Build history of the part. All positions in model axes, mm. Face numbers are marked on the shaded views. A direction names the side the tool comes from. Round coordinates to 2 decimals unless told otherwise and drop trailing zeros. Loops run counter-clockwise (first coordinate to the right, second up) from the corner with the lowest first, then second, coordinate; pieces in that order, holes last.
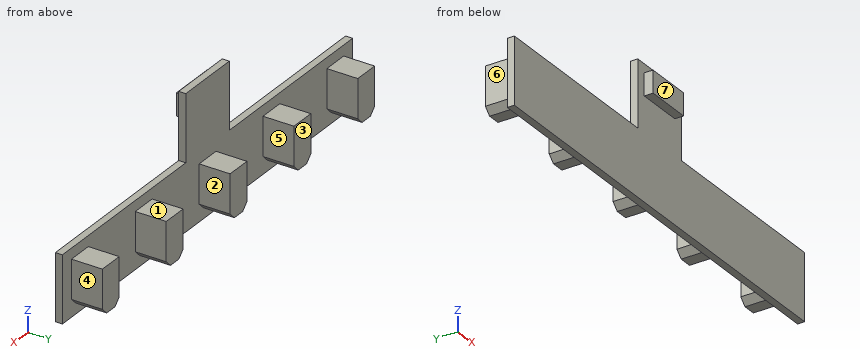
from build123d import *

# Parameters (mm, degrees)
SKETCH1_W           = 15
SKETCH1_H           = 15
SKETCH1_W_2         = 10.56
SKETCH1_H_2         = 5
BOSS_EXTRUDE1_DEPTH = 1.6
SKETCH1_3_W         = 10.56
SKETCH1_3_H         = 5
BOSS_EXTRUDE2_DEPTH = 2
BOSS_EXTRUDE3_DEPTH = 8.6


with BuildPart() as part:
    # Sketch1 → Boss-Extrude1 (new body)
    # profile 1 of 3: a face of its own
    with BuildSketch(Plane(origin=(0, 0, 0), x_dir=(1, 0, 0), z_dir=(0, 1, 0))):
        with Locations((0, 3)):
            Rectangle(SKETCH1_W, SKETCH1_H)
        Rectangle(SKETCH1_W_2, SKETCH1_H_2, mode=Mode.SUBTRACT)
    # profile 2 of 3: a face of its own
    with BuildSketch(Plane(origin=(0, 0, 0), x_dir=(1, 0, 0), z_dir=(0, 1, 0))):
        Rectangle(SKETCH1_W_2, SKETCH1_H_2)
    # profile 3 of 3: a face of its own
    with BuildSketch(Plane(origin=(0, 0, 0), x_dir=(1, 0, 0), z_dir=(0, 1, 0))):
        Polygon((-50, 10.5), (-7.5, 10.5), (7.5, 10.5), (50, 10.5), (50, 25.5), (-50, 25.5), align=None)
        Polygon((-42.569302237, 23.1), (-41.1, 21.630697763), (-41.1, 12.9), (-46.9, 12.9), (-46.9, 21.630697763), (-45.430697763, 23.1), align=None, mode=Mode.SUBTRACT)
        Polygon((-20.569302237, 23.1), (-19.1, 21.630697763), (-19.1, 12.9), (-24.9, 12.9), (-24.9, 21.630697763), (-23.430697763, 23.1), align=None, mode=Mode.SUBTRACT)
        Polygon((2.9, 12.9), (-2.9, 12.9), (-2.9, 21.630697763), (-1.430697763, 23.1), (1.430697763, 23.1), (2.9, 21.630697763), align=None, mode=Mode.SUBTRACT)
        Polygon((23.430697763, 23.1), (24.9, 21.630697763), (24.9, 12.9), (19.1, 12.9), (19.1, 21.630697763), (20.569302237, 23.1), align=None, mode=Mode.SUBTRACT)
        Polygon((45.430697763, 23.1), (46.9, 21.630697763), (46.9, 12.9), (41.1, 12.9), (41.1, 21.630697763), (42.569302237, 23.1), align=None, mode=Mode.SUBTRACT)
    extrude(amount=BOSS_EXTRUDE1_DEPTH)

    # Sketch1_3 → Boss-Extrude2 (add)
    with BuildSketch(Plane(origin=(0, 0, 0), x_dir=(1, 0, 0), z_dir=(0, 1, 0))):
        Rectangle(SKETCH1_3_W, SKETCH1_3_H)
    extrude(amount=-BOSS_EXTRUDE2_DEPTH)

    # Sketch1_4 → Boss-Extrude3 (add)
    with BuildSketch(Plane(origin=(0, 0, 0), x_dir=(1, 0, 0), z_dir=(0, 1, 0))):
        Polygon((23.430697763, 23.1), (24.9, 21.630697763), (24.9, 12.9), (19.1, 12.9), (19.1, 21.630697763), (20.569302237, 23.1), align=None)
        Polygon((45.430697763, 23.1), (46.9, 21.630697763), (46.9, 12.9), (41.1, 12.9), (41.1, 21.630697763), (42.569302237, 23.1), align=None)
        Polygon((2.9, 21.630697763), (2.9, 12.9), (-2.9, 12.9), (-2.9, 21.630697763), (-1.430697763, 23.1), (1.430697763, 23.1), align=None)
        Polygon((-20.569302237, 23.1), (-19.1, 21.630697763), (-19.1, 12.9), (-24.9, 12.9), (-24.9, 21.630697763), (-23.430697763, 23.1), align=None)
        Polygon((-42.569302237, 23.1), (-41.1, 21.630697763), (-41.1, 12.9), (-46.9, 12.9), (-46.9, 21.630697763), (-45.430697763, 23.1), align=None)
    extrude(amount=BOSS_EXTRUDE3_DEPTH)


solid = part.part
(1) Which spindle directions (+Z, -Z, +X, -X, +Y, -Y) get a long thin tool onto all of the face, cutting with end or side? Do the marked faces 1, 2 and 3. Say none if no direction does.
Responses:
face 1: +Z, +X, -X, +Y
face 2: +Z, -Z, +Y
face 3: +Z, -Z, +X, -X, +Y
(2) Probe line 1 (X direction, y = 2.75, z = -14.25); line 2 (X direction, y = 7.5, z = -22.5); line 3 (Y direction, x = 11, z = -11.75). List the from-to ranges inside material, lowest first.
Responses:
line 1: x = -46.9 to -41.1, -24.9 to -19.1, -2.9 to 2.9, 19.1 to 24.9, 41.1 to 46.9
line 2: x = -46.03 to -41.97, -24.03 to -19.97, -2.03 to 2.03, 19.97 to 24.03, 41.97 to 46.03
line 3: y = 0 to 1.6
(3) Slice it at C-C on y = -1. List the corners of the cut face in (x, z), plus the area to 3 significant figures.
Responses:
outline: (-5.28, -2.5) - (5.28, -2.5) - (5.28, 2.5) - (-5.28, 2.5) - close
area: 52.8 mm2
(4) Slice it at B-B on z = -15.5. List the corners of the cut face in (x, y).
Responses:
outline: (-50, 0) - (50, 0) - (50, 1.6) - (46.9, 1.6) - (46.9, 8.6) - (41.1, 8.6) - (41.1, 1.6) - (24.9, 1.6) - (24.9, 8.6) - (19.1, 8.6) - (19.1, 1.6) - (2.9, 1.6) - (2.9, 8.6) - (-2.9, 8.6) - (-2.9, 1.6) - (-19.1, 1.6) - (-19.1, 8.6) - (-24.9, 8.6) - (-24.9, 1.6) - (-41.1, 1.6) - (-41.1, 8.6) - (-46.9, 8.6) - (-46.9, 1.6) - (-50, 1.6) - close
(5) Slice it at D-D on x = -30. List the corners of the cut face in (y, z), plus the area to 3 significant figures.
Responses:
outline: (0, -25.5) - (1.6, -25.5) - (1.6, -10.5) - (0, -10.5) - close
area: 24.0 mm2
(6) Pull direction X, two halves, no side cores. Call the marked faces 4, 5, 6 and 7: +X half, -X half, draft (parallel to the pull), parting line (faces both ways), or undercut.
Responses:
face 4: +X half
face 5: undercut
face 6: -X half
face 7: draft
(7) Pin check, flat tips, straight feed: P1, Ø3, axis at x = -43.5, y = 4.5, coming from the +Z side; P2, Ø5.5, axis at y = 6.5, z = -15, coming from the +X side; P3, Ø1.3, axis at y = 0.5, z = 0, coming from the -X side. Stop position of each tip, or through.
Responses:
P1: stops at z = -12.9
P2: stops at x = 46.9
P3: stops at x = -7.5
(8) Slice it at A-A on y = 4.5. Count the separate pieces of the cut face and the enclosed holes in it, plus the area to 3 significant figures.
Responses:
separate pieces: 5
enclosed holes: 0
area: 285 mm2
